from build123d import *

# Parameters (mm, degrees)
SKETCH1_W           = 50
SKETCH1_H           = 20
BOSS_EXTRUDE1_DEPTH = 2
SKETCH2_W           = 2
SKETCH2_H           = 20
BOSS_EXTRUDE2_DEPTH = 30
SKETCH4_W           = 9.955385113
SKETCH4_H           = 6.56478527
BOSS_EXTRUDE3_DEPTH = 7
CUT_EXTRUDE1_DEPTH  = 7
SKETCH6_R           = 1.5
CUT_EXTRUDE2_DEPTH  = 7
SKETCH7_R           = 1.5
CUT_EXTRUDE3_DEPTH  = 7


with BuildPart() as part:
    # Sketch1 → Boss-Extrude1 (new body)
    with BuildSketch(Plane(origin=(0, 0, 0), x_dir=(1, 0, 0), z_dir=(0, 1, 0))):
        with Locations((25, 10)):
            Rectangle(SKETCH1_W, SKETCH1_H)
    extrude(amount=BOSS_EXTRUDE1_DEPTH)

    # Sketch2 → Boss-Extrude2 (add)
    with BuildSketch(Plane(origin=(0, 2, 0), x_dir=(1, 0, 0), z_dir=(0, 1, 0))):
        with Locations((1, 10)):
            Rectangle(SKETCH2_W, SKETCH2_H)
    extrude(amount=BOSS_EXTRUDE2_DEPTH)

    # Sketch4 → Boss-Extrude3 (add)
    with BuildSketch(Plane(origin=(0, 2, 0), x_dir=(1, 0, 0), z_dir=(0, 1, 0))):
        with Locations((6.977692557, 10.002392635)):
            Rectangle(SKETCH4_W, SKETCH4_H)
    extrude(amount=BOSS_EXTRUDE3_DEPTH)

    # Sketch5 → Cut-Extrude1 (cut)
    with BuildSketch(Plane.XY.offset(-6.72)):
        Polygon((2, 9), (11.955385113, 2), (11.955385113, 9), align=None)
    extrude(amount=-CUT_EXTRUDE1_DEPTH, mode=Mode.SUBTRACT)

    # Sketch6 → Cut-Extrude2 (cut)
    with BuildSketch(Plane(origin=(0, 2, 0), x_dir=(1, 0, 0), z_dir=(0, 1, 0))):
        with Locations(Location((23.955385113, 10, 0), (0, 0, 270))):
            Circle(SKETCH6_R)
        with Locations(Location((35.955385113, 10, 0), (0, 0, 270))):
            Circle(SKETCH6_R)
    extrude(amount=-CUT_EXTRUDE2_DEPTH, mode=Mode.SUBTRACT)

    # Sketch7 → Cut-Extrude3 (cut)
    with BuildSketch(Plane(origin=(2, 0, 0), x_dir=(0, 0, -1), z_dir=(1, 0, 0))):
        with Locations((10.001560414, 17)):
            Circle(SKETCH7_R)
        with Locations((10.000728193, 24.999999957)):
            Circle(SKETCH7_R)
    extrude(amount=-CUT_EXTRUDE3_DEPTH, mode=Mode.SUBTRACT)


solid = part.part
Work out the finished part from the listing and answer in its coordinate system (mm). A direction names the side the tool comes from. Round coordinates to 2 decimals unless told otherwise and drop trailing zeros. Order: outer loops, then holes, each group sorted by start corner. A loop starts at its lowest first (then second) coordinate and runs counter-clockwise, first axis right, second up. Notation, with made-up numbers: M 73.5,43 L 116.5,43 A3 ccw 116.5,47 Z; hole C 12.25,5.25 d1. An arc over 180 degrees is marked long. One line per item, written item: value.
Q1. Find section A-A on z = -10. Write down the section's boundary in (x, y), then the cut area to 3 significant figures.
Derived:
outline: M 0,0 L 22.46,0 L 22.46,2 L 11.96,2 L 2,9 L 2,15.5 L 0,15.5 Z; M 0,18.5 L 2,18.5 L 2,23.5 L 0,23.5 Z; M 0,26.5 L 2,26.5 L 2,32 L 0,32 Z; M 25.46,0 L 34.46,0 L 34.46,2 L 25.46,2 Z; M 37.46,0 L 50,0 L 50,2 L 37.46,2 Z
area: 171 mm²
Q2. Find section D-D on z = -6. Write down the section's boundary in (x, y), then the cut area to 3 significant figures.
Derived:
outline: M 0,0 L 50,0 L 50,2 L 2,2 L 2,32 L 0,32 Z
area: 160 mm²
Q3. Flat-ended cylindrical pins translate along their axes: pin 1 (2 mm diameter, centred on x = 7, y = 5, fed in from +Z); pin 2 (3 mm diameter, centred on y = 24.5, z = -16.5, fed in from +X); pin 3 (3.5 mm diameter, centred on x = 23.96, z = -10, fed in from +Y). Find the tip coordinate at first contact, or state that the pin passes through.
Derived:
pin 1: z = -6.72
pin 2: x = 2
pin 3: y = 2
Q4. Straight lines are drawn through the part: line 1 (X direction, y = 1.3, z = -10); line 2 (Y direction, x = 47, z = -18.5); line 3 (Z direction, x = 0.45, y = 25). For each, find the intervals that lie inside material, in ascending order.
Derived:
line 1: 0 to 22.46, 25.46 to 34.46, 37.46 to 50
line 2: 0 to 2
line 3: -20 to -11.5, -8.5 to 0
Q5. Determine the mould class of faces 1 (the face through (1, 32, -10)), 2 (the face through (1.014, 26.487, -9.805)), 3 (the face through (6, 5, -6.72)) for opening direction Y: released by +Y, released by -Y, zero draft, split by the parting line, or undercut.
Derived:
face 1: released by +Y
face 2: undercut
face 3: zero draft
Q6. Find section C-C on x = 9. Write down the section's boundary in (y, z).
Derived:
outline: M 0,-20 L 2,-20 L 2,-13.28 L 4.08,-13.28 L 4.08,-6.72 L 2,-6.72 L 2,0 L 0,0 Z
Q7. Find section B-B on y = 25. Write down the section's boundary in (x, z).
Derived:
outline: M 0,-20 L 2,-20 L 2,-11.5 L 0,-11.5 Z; M 0,-8.5 L 2,-8.5 L 2,0 L 0,0 Z
Q8. For faces 4 (the face through (6, 5, -13.285)), 5 (the face through (1.014, 18.014, -8.896)), determine the directions among +Z, -Z, +X, -X, +Y, -Y from which every point of the face is accessible in a straight line to the end or side of a thin tool.
Derived:
face 4: -Z, +X, +Y
face 5: +X, -X
